Input: part model. Units: mm. Frame: model coordinates. Give positions to 0.01 mm unless a question says otherwise; leave off trailing zeros. Loops run counter-clockwise (first coordinate to the right, second up) from the corner with the lowest first, then second, coordinate; pieces in that order, holes last. Notation, with made-up numbers: M 87.5,23 L 141.5,23 A34 ccw 141.5,59 Z; hole C 17,-13.75 d8. An arc over 180 degrees is marked long. Answer as a JSON object with one key per item and string values. Group by question number.
1) Ray query, L1, parallel to Y at x = -18, z = 0; L2, parallel to Z at x = -16, y = -0.25; L3, parallel to Z at x = -34.5, y = 0.55. Return the intervals inside material, ascending.
2) Section query C-C on x = 9. Return loops of the section in (y, z), plus the area to 3 significant figures.
3) Section query A-A on y = 0. Return loops of the section in (x, z).
4) Draft query along Y for faces 1 (the cylindrical face through (0.66, 0.83, -0.18)), 2 (the flat face through (1, -2, 0)), 3 (the flat face through (1, 0, -2)). Return one class per face: +Y half, -Y half, draft (parallel to the pull), parting line (faces both ways), or undercut.
from build123d import *

# Parameters (mm, degrees)
ESBO_O1_W                         = 4
ESBO_O1_H                         = 4
RESSALTO_EXTRUS_O1_DEPTH          = 47.5
CORTE_EXTRUS_O1_REACH             = 97.042
ESBO_O2_R                         = 0.85
CORTE_EXTRUS_O1_DIRECTION_2_DEPTH = 96.042095936


with BuildPart() as part:
    # Esboço1 → Ressalto-extrusão1 (new, symmetric)
    with BuildSketch(Plane(origin=(0, 0, 0), x_dir=(0, 0, -1), z_dir=(1, 0, 0))):
        Rectangle(ESBO_O1_W, ESBO_O1_H)
    extrude(amount=RESSALTO_EXTRUS_O1_DEPTH, both=True)

    # Esboço2 → Corte-extrusão1 (cut, up to next)
    with BuildSketch(Plane(origin=(47.5, 0, 0), x_dir=(0, 0, -1), z_dir=(1, 0, 0)), mode=Mode.PRIVATE) as corte_extrus_o1_sk1:
        with Locations(Location((0, 0, 0), (0, 0, 180))):
            Circle(ESBO_O2_R)
    corte_extrus_o1_tool1 = extrude(corte_extrus_o1_sk1.sketch, amount=-CORTE_EXTRUS_O1_REACH, mode=Mode.PRIVATE) & part.part
    add(corte_extrus_o1_tool1.solids().sort_by_distance((47.5, 0, 0))[0], mode=Mode.SUBTRACT)

    # Esboço2 → Corte-extrusão1 direction 2 (cut)
    with BuildSketch(Plane(origin=(47.5, 0, 0), x_dir=(0, 0, -1), z_dir=(1, 0, 0))):
        with Locations(Location((0, 0, 0), (0, 0, 180))):
            Circle(ESBO_O2_R)
    extrude(amount=CORTE_EXTRUS_O1_DIRECTION_2_DEPTH, mode=Mode.SUBTRACT)


solid = part.part
Output:
{
 "1": {"L1": "y = -2 to -0.85, 0.85 to 2", "L2": "z = -2 to -0.81, 0.81 to 2", "L3": "z = -2 to -0.65, 0.65 to 2"},
 "2": {"outline": "M -2,-2 L 2,-2 L 2,2 L -2,2 Z; hole C 0,0 d1.7", "area": "13.7 mm^2"},
 "3": {"outline": "M -47.5,-2 L 47.5,-2 L 47.5,-0.85 L -47.5,-0.85 Z; M -47.5,0.85 L 47.5,0.85 L 47.5,2 L -47.5,2 Z"},
 "4": {"face 1": "undercut", "face 2": "-Y half", "face 3": "draft"}
}
